Can you work these out from the model? Positions are in its coordinate system, mm. Give positions to 0.01 mm unless a question says otherwise; leave off trailing zeros. Loops run counter-clockwise (first coordinate to the right, second up) from the corner with the lowest first, then second, coordinate; pieces in that order, holes last. Notation, with made-up numbers: (-11, -39) -> (16, -39) arc R29 cw to (16, -10) -> close; hole circle Ø9 at (83, -35). An arc over 180 degrees is marked (long way). Use CSV: the item, a comma, the result in double quotes.
from build123d import *

# Parameters (mm, degrees)
SKETCH2_R            = 17.5
BOSS_EXTRUDE1_DEPTH  = 20
CUT_SWEEP1_PROFILE_R = 1
SKETCH62_R           = 2.5
CUT_EXTRUDE3_DEPTH   = 32.819805153
SKETCH65_R           = 6
CUT_EXTRUDE4_DEPTH   = 11


with BuildPart() as part:
    # Sketch2 → Boss-Extrude1 (new body)
    with BuildSketch(Plane(origin=(0, 0, 0), x_dir=(1, 0, 0), z_dir=(0, 1, 0))):
        with Locations(Location((0, 0, 0), (0, 0, 270))):
            Circle(SKETCH2_R)
    extrude(amount=BOSS_EXTRUDE1_DEPTH)

    # Cut-Sweep1: sweep along a path in Sketch39
    with BuildLine(Plane(origin=(0, 20, 0), x_dir=(1, 0, 0), z_dir=(0, 1, 0))) as cut_sweep1_path:
        CenterArc((0, 0), 9, 0, 360)
    # Cut-Sweep1 profile (on start of the path) → Cut-Sweep1 (sweep, cut)
    with BuildSketch(Plane(origin=(9, 20, 0), x_dir=(-1, 0, 0), z_dir=(0, 0, -1))):
        Circle(CUT_SWEEP1_PROFILE_R)
    sweep(path=cut_sweep1_path.line, mode=Mode.SUBTRACT)

    # Sketch62 → Cut-Extrude3 (cut, through all)
    with BuildSketch(Plane(origin=(0, 0, 0), x_dir=(1, 0, 0), z_dir=(0, 1, 0))):
        with Locations(Location((0, 0, 0), (0, 0, 270))):
            Circle(SKETCH62_R)
    extrude(amount=CUT_EXTRUDE3_DEPTH, mode=Mode.SUBTRACT)

    # Sketch65 → Cut-Extrude4 (cut)
    with BuildSketch(Plane(origin=(0, 20, 0), x_dir=(1, 0, 0), z_dir=(0, 1, 0))):
        with Locations(Location((0, 0, 0), (0, 0, 270))):
            Circle(SKETCH65_R)
    extrude(amount=-CUT_EXTRUDE4_DEPTH, mode=Mode.SUBTRACT)


solid = part.part
(1) If we section it at C-C, the plane y = 3: Write out the boundary of the cut face in (x, z), then the cut area to 3 significant figures.
Answer sheet:
outline,"circle Ø35 at (0, 0); hole circle Ø5 at (0, 0)"
area,"942 mm2"
(2) If we section it at A-A, the plane x = 0: Write out the boundary of the cut face in (y, z).
Answer sheet:
outline,"(0, -17.5) -> (20, -17.5) -> (20, -10) arc R1 cw to (20, -8) -> (20, -6) -> (9, -6) -> (9, -2.5) -> (0, -2.5) -> close; (0, 2.5) -> (9, 2.5) -> (9, 6) -> (20, 6) -> (20, 8) arc R1 cw to (20, 10) -> (20, 17.5) -> (0, 17.5) -> close"
(3) Will these pins go through, and if not, where does the flat tip stop? pin 1 Ø12 at (x, y) = (-7, 8) entering from -Z; pin 2 Ø4 at (x, z) = (-4, 4) entering from -Y; pin 3 Ø6 at (x, z) = (-2.5, 0) entering from +Y; pin 4 Ø10 at (y, z) = (7.5, -6.5) entering from -X.
Answer sheet:
pin 1,"stops at z = -17.47"
pin 2,"stops at y = 0"
pin 3,"stops at y = 9"
pin 4,"stops at x = -17.44"
(4) If I drill on L1, parallel to X at y = 10.5, z = 0; L2, parallel to X at y = 6.75, z = 0; L3, parallel to Z at x = 2.5, y = 18.5, over which ranges is the centre line in solid material (lowest first)? Write a range as from..to.
Answer sheet:
L1,"x = -17.5..-6, 6..17.5"
L2,"x = -17.5..-2.5, 2.5..17.5"
L3,"z = -17.32..-5.45, 5.45..17.32"
(5) If we section it at D-D, the plane z = 12.5: Write out the boundary of the cut face in (x, y), then the cut area to 3 significant figures.
Answer sheet:
outline,"(-12.25, 0) -> (12.25, 0) -> (12.25, 20) -> (-12.25, 20) -> close"
area,"490 mm2"
(6) We'd pull the mould along Z, two halves only. Please class faces 1 (the face through (-8, 20, 8)), 2 (the face through (1.802, 14.577, 5.723)), 3 (the face through (-10.648, 9.86, -13.887)), 4 (the face through (0, 9, 3)): released by +Z, released by -Z, zero draft, split by the parting line, or undercut.
Answer sheet:
face 1,"zero draft"
face 2,"undercut"
face 3,"split by the parting line"
face 4,"undercut"
(7) If we section it at B-B, the plane z = 0: Write out the boundary of the cut face in (x, y).
Answer sheet:
outline,"(-17.5, 0) -> (-2.5, 0) -> (-2.5, 9) -> (-6, 9) -> (-6, 20) -> (-8, 20) arc R1 cw to (-10, 20) -> (-17.5, 20) -> close; (2.5, 0) -> (17.5, 0) -> (17.5, 20) -> (10, 20) arc R1 cw to (8, 20) -> (6, 20) -> (6, 9) -> (2.5, 9) -> close"
